from build123d import *

# Parameters (mm, degrees)
SKETCH1_W           = 2
SKETCH1_H           = 7.2
SKETCH1_W_2         = 18
BOSS_EXTRUDE3_DEPTH = 15
BOSS_EXTRUDE4_START = 15
SKETCH1_4_W         = 2
SKETCH1_4_H         = 7.2
BOSS_EXTRUDE4_DEPTH = 8.5
BOSS_EXTRUDE5_START = -3.6
SKETCH3_W           = 2
SKETCH3_H           = 3
BOSS_EXTRUDE5_DEPTH = 7.2


with BuildPart() as part:
    # Sketch1 → Boss-Extrude3 (new body)
    with BuildSketch(Plane.XY):
        Polygon((9, 3.6), (11, 3.6), (11, 5.6), (-11, 5.6), (-11, 3.6), (-9, 3.6), align=None)
        with Locations((-10, 0)):
            Rectangle(SKETCH1_W, SKETCH1_H)
        Rectangle(SKETCH1_W_2, SKETCH1_H)
        Polygon((11, -3.6), (11, -5.6), (-11, -5.6), (-11, -3.6), (-9, -3.6), (9, -3.6), align=None)
        with Locations((10, 0)):
            Rectangle(SKETCH1_W, SKETCH1_H)
    extrude(amount=BOSS_EXTRUDE3_DEPTH)

    # Sketch1<4> → Boss-Extrude4 (add)
    with BuildSketch(Plane.XY.offset(BOSS_EXTRUDE4_START)):
        with Locations((-10, 0)):
            Rectangle(SKETCH1_4_W, SKETCH1_4_H)
        with Locations((10, 0)):
            Rectangle(SKETCH1_4_W, SKETCH1_4_H)
    extrude(amount=BOSS_EXTRUDE4_DEPTH)

    # Sketch3 → Boss-Extrude5 (add)
    with BuildSketch(Plane(origin=(0, 0, 0), x_dir=(1, 0, 0), z_dir=(0, 1, 0)).offset(BOSS_EXTRUDE5_START)):
        with Locations((-10, -25)):
            Rectangle(SKETCH3_W, SKETCH3_H)
        with BuildLine():
            Line((-9, -23.5), (-9, -26.5))
            ThreePointArc((-9, -26.5), (-7.5, -25), (-9, -23.5))
        make_face()
    boss_extrude5 = extrude(amount=BOSS_EXTRUDE5_DEPTH)

    # Mirror1: Boss-Extrude5 across plane
    add(boss_extrude5.mirror(Plane(origin=(0, 0, 0), x_dir=(0, 0, 1), z_dir=(1, 0, 0))))


solid = part.part
Source: CAD feature listing. Evaluate the final solid. Frame: model axes, mm. A direction names the side the tool comes from. Round coordinates to 2 decimals unless told otherwise and drop trailing zeros. Write each loop counter-clockwise with the first axis right and the second up, starting at its lowest first coordinate (ties: lowest second). Pieces come first, ordered by that corner, then holes. Notation, with made-up numbers: (-1.5, 69.5) - (5.5, 69.5) arc R11 ccw to (5.5, 79.5) - close; hole circle Ø4 at (0.5, 7.25). An arc over 180 degrees is marked (long way). Use CSV: the item, a comma, the result in double quotes. Start each with the question number.
(1) Mould query, pull axis Z, two halves, no side actions, for faces 1 (the face through (0, 0, 0)), 2 (the face through (-9, 0, 19)), 3 (the face through (-10, 0, 26.5)). Classes: pulls with the +Z half, pulls with the -Z half, needs draft (parallel to the pull), parting line crosses it, or undercut.
(2) Cut plane B-B, the plane y = -2. Return loops of the section in (x, z).
(3) First-contact query: pin 1 Ø5.5 at (x, y) = (-0.5, 3) entering from +Z; pin 2 Ø4 at (x, z) = (-8.5, 18.5) entering from -Y; pin 3 Ø4 at (x, z) = (9, 19.5) entering from +Y. Flat tips, straight axial feed; report the tip coordinate or a pass-through.
(4) Set-up query: faces 4 (the face through (10, 3.6, 21)), 5 (the face through (7.5, -0.1, 25)), 6 (the face through (-10, -3.6, 21)). Return all of +Z, -Z, +X, -X, +Y, -Y with unobstructed straight access to the full face (end or side cutting, diameter ignored); none if empty.
(5) Cut plane D-D, the plane y = -5. Return loops of the section in (x, z).
(6) Cut plane A-A, the plane z = 25. Return loops of the section in (x, y), and give its area (3 significant figures).
(7) Cut plane C-C, the plane x = -5.75. Return loops of the section in (y, z), and give its area (3 significant figures).
(8) Material intervals for probe 1 along Z at (x, y) = (9.25, -4.5); probe 2 along X at (y, z) = (-3.25, 16.75); probe 3 along Y at (x, z) = (-9.75, 16.5), sorted ascending. Write a range as [from, to].
Geometry says:
1,face 1,"pulls with the -Z half"
1,face 2,"undercut"
1,face 3,"pulls with the +Z half"
2,outline,"(-11, 0) - (11, 0) - (11, 26.5) - (9, 26.5) arc R1.5 ccw to (9, 23.5) - (9, 15) - (-9, 15) - (-9, 23.5) arc R1.5 ccw to (-9, 26.5) - (-11, 26.5) - close"
3,pin 1,"z = 15"
3,pin 2,"y = -3.6"
3,pin 3,"y = 3.6"
4,face 4,"+Z, +X, -X, +Y"
4,face 5,"+Y, -Y"
4,face 6,"+Z, +X, -X, -Y"
5,outline,"(-11, 0) - (11, 0) - (11, 15) - (-11, 15) - close"
6,outline,"(-11, -3.6) - (-7.5, -3.6) - (-7.5, 3.6) - (-11, 3.6) - close; (7.5, -3.6) - (11, -3.6) - (11, 3.6) - (7.5, 3.6) - close"
6,area,"50.4 mm²"
7,outline,"(-5.6, 0) - (5.6, 0) - (5.6, 15) - (-5.6, 15) - close"
7,area,"168 mm²"
8,probe 1,"[0, 15]"
8,probe 2,"[-11, -9], [9, 11]"
8,probe 3,"[-3.6, 3.6]"
